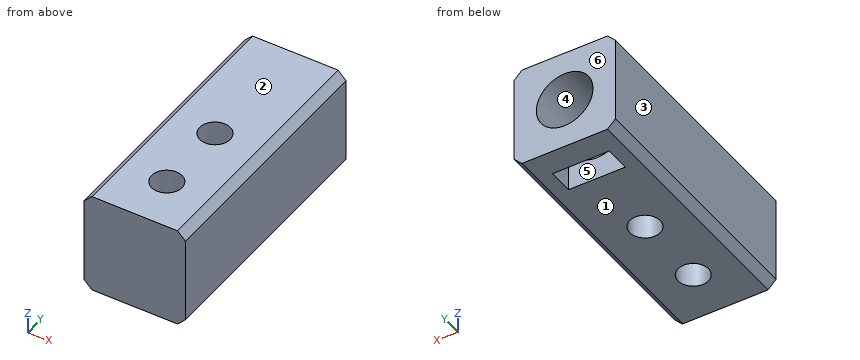
Autodesk Inventor part; units mm, degrees
ref_plane "YZ Plane" through (0, 0, 0) normal (1, 0, 0) x (0, 1, 0)
ref_plane "XZ Plane" through (0, 0, 0) normal (0, 1, 0) x (-1, 0, 0)
ref_plane "XY Plane" through (0, 0, 0) normal (0, 0, 1) x (1, 0, 0)
sketch "Sketch1" plane through (0, 0, 0) normal (0, 1, 0) x (-1, 0, 0)
  line L0 (0, 0) -> (40, 0)
  line L1 (40, 0) -> (40, -40)
  line L2 (40, -40) -> (0, -40)
  line L3 (0, -40) -> (0, 0)
  dimension "d0" = 40
  dimension "d1" = 40
extrude "Extrusion1" add sketch "Sketch1" along normal blind 100
sketch "Sketch2" plane through (-40, 0, 0) normal (0, 0, 1) x (1, 0, 0)
  circle A0 centre (20, 20) radius 6
  circle A1 centre (20, 50) radius 6
  line L0 (40, 0) -> (0, 0)
  line L1 (0, 0) -> (0, 100)
  dimension "d4" = 12
  dimension "d5" = 12
  dimension "d6" = 20
  dimension "d7" = 30
  dimension "d8" = 20
  dimension "d9" = 20
extrude "Extrusion2" cut sketch "Sketch2" against normal blind 40
sketch "Sketch3" plane through (0, 100, 0) normal (0, 1, 0) x (1, 0, 0)
  circle A0 centre (-20, 20) radius 11.15
  line L0 (-40, 40) -> (-40, 0)
  line L1 (-40, 0) -> (0, 0)
  dimension "d12" = 22.3
  dimension "d13" = 20
  dimension "d14" = 20
extrude "Extrusion3" cut sketch "Sketch3" against normal blind 30
sketch "Sketch4" plane through (0, 0, -40) normal (0, 0, -1) x (-1, 0, 0)
  line L0 (8.85, 90) -> (31.15, 90)
  line L1 (31.15, 90) -> (31.15, 80)
  line L2 (31.15, 80) -> (8.85, 80)
  line L3 (8.85, 80) -> (8.85, 90)
  line L4 (8.85, 90) -> (31.15, 80) construction
  line L5 (31.15, 90) -> (8.85, 80) construction
  line L6 (0, 0) -> (0, 100)
  line L7 (0, 100) -> (40, 100)
  point P0 (20, 85)
  dimension "d17" = 22.3
  dimension "d18" = 10
  dimension "d19" = 20
  dimension "d20" = 15
extrude "Extrusion4" cut sketch "Sketch4" against normal blind 20
chamfer "Chamfer1" distance 3.175 angle 45 4 edges at (-40, 50, 0) (-40, 50, -40) (0, 50, -40) (0, 50, 0)
properties part number "simplifiedY"
Verification items for the finished model (mm, model axes). Face numbers are marked on the shaded views. A direction names the side the tool comes from. Coordinates: 2 decimals unless noted, no trailing zeros. Write each loop counter-clockwise with the first axis right and the second up, starting at its lowest first coordinate (ties: lowest second). Pieces come first, ordered by that corner, then holes. Notation, with made-up numbers: M 85,15.5 L 114,15.5 A23 cw 114,30.5 Z; hole C 27,-12 d9. An arc over 180 degrees is marked long. One line per item, written item: value.
Item 1: Mould release check, pull along Z, two halves, no side actions. Record for the marked faces 1, 2, 3 and 4: pulls with the +Z half, pulls with the -Z half, needs draft (parallel to the pull), parting line crosses it, or undercut.
Check sheet entries:
face 1: pulls with the -Z half
face 2: pulls with the +Z half
face 3: needs draft
face 4: undercut
Item 2: Access from +Z, -Z, +X, -X, +Y, -Y to the whole of each face (thin tool, end or side, straight path). Record for the marked faces 5 and 6.
Check sheet entries:
face 5: -Z
face 6: +Z, -Z, +X, -X, +Y
Item 3: Scan lines: line 1 along Y through (x, z) = (-20, -29); line 2 along Y through (x, z) = (-15.5, -21); line 3 along X through (y, z) = (77, -20). Record each from-to range of solid material in increasing order.
Check sheet entries:
line 1: y = 0 to 14, 26 to 44, 56 to 70
line 2: y = 0 to 16.03, 23.97 to 46.03, 53.97 to 70
line 3: x = -40 to -31.15, -8.85 to 0
Item 4: Section check C-C, the plane y = 50. Record the boundary of the cut face in (x, z) (3 decimals), plus the area to 3 significant figures.
Check sheet entries:
outline: M -40,-36.825 L -36.825,-40 L -26,-40 L -26,0 L -36.825,0 L -40,-3.175 Z; M -14,-40 L -3.175,-40 L 0,-36.825 L 0,-3.175 L -3.175,0 L -14,0 Z
area: 1,100 mm^2
Item 5: Section check B-B, the plane z = -6. Record the boundary of the cut face in (x, y).
Check sheet entries:
outline: M -40,0 L 0,0 L 0,100 L -40,100 Z; hole C -20,20 d12; hole C -20,50 d12
Item 6: Section check A-A, the plane x = -20. Record the boundary of the cut face in (y, z), plus the area to 3 significant figures.
Check sheet entries:
outline: M 0,-40 L 14,-40 L 14,0 L 0,0 Z; M 26,-40 L 44,-40 L 44,0 L 26,0 Z; M 56,-40 L 80,-40 L 80,-31.15 L 70,-31.15 L 70,-8.85 L 100,-8.85 L 100,0 L 56,0 Z; M 90,-40 L 100,-40 L 100,-31.15 L 90,-31.15 Z
area: 2,280 mm^2
Item 7: Gauge pin test, flat ends, axial feed: pin 1 Ø2 at (x, z) = (-25, -19) entering from +Y; pin 2 Ø9.5 at (x, y) = (-20, 20) entering from -Z. Record the tip position at first contact, or that the pin passes through.
Check sheet entries:
pin 1: stops at y = 70
pin 2: passes through
Item 8: Section check D-D, the plane z = -17. Record the boundary of the cut face in (x, y).
Check sheet entries:
outline: M -40,0 L 0,0 L 0,100 L -9.26,100 L -9.26,70 L -30.74,70 L -30.74,100 L -40,100 Z; hole C -20,20 d12; hole C -20,50 d12
